Part model, mm, in its own coordinate system. Coordinates: 2 decimals unless noted, no trailing zeros. Order: outer loops, then holes, each group sorted by start corner. A loop starts at its lowest first (then second) coordinate and runs counter-clockwise, first axis right, second up.
1) Cut at B-B (y = 3.25). List the corners of the cut face in (x, z), and give its area (3 significant figures).
2) Cut at C-C (z = 45). Give the number of separate pieces and of enclosed holes in the cut face, and give its area (3 significant figures).
3) Wall check: L1, parallel to Y at x = 210.5, z = 0; L2, parallel to X at y = -0.5, z = 27.5. Give the ranges that are in metal, low to high.
4) Pin check, flat tips, straight feed: pin 1 Ø8 at (x, y) = (311.5, -3.5) entering from +Z; pin 2 Ø5 at (y, z) = (7.5, 44) entering from +X; pin 3 Ø6 at (x, y) = (398, -5.5) entering from -Z. Stop position of each tip, or through.
5) Cut at A-A (x = 258.5). List the corners of the cut face in (y, z), and give its area (3 significant figures).
Autodesk Inventor part; units mm, degrees
ref_plane "YZ Plane" through (0, 0, 0) normal (1, 0, 0) x (0, 1, 0)
ref_plane "XZ Plane" through (0, 0, 0) normal (0, 1, 0) x (-1, 0, 0)
ref_plane "XY Plane" through (0, 0, 0) normal (0, 0, 1) x (1, 0, 0)
sketch "Szkic1" plane through (0, 0, 0) normal (1, 0, 0) x (0, 1, 0)
  circle A0 centre (0, 0) radius 10
  dimension "d0" = 20
extrude "Wyciągnięcie proste1" add sketch "Szkic1" along normal blind 475
shell "Skorupa1" thickness 2 removed faces 2 at (475, -1.182, 3.1167) at (0, -1.182, 3.1167)
sketch "Szkic2" plane through (0, 0, 0) normal (0, 0, 1) x (1, 0, 0)
  line L0 (100, 28.3712) -> (100, -25.6691)
  line L1 (0, 10) -> (0, -10)
  point P0 (0, 0)
  dimension "d4" = 100
bend part "Gięcie części1" radius 50.9296 angle 45 line through (100, 28.3712, 0) along (0, -1, 0) centre toward (0, 0, 1) moving side (-1, 0, 0) both sides no
sketch "Szkic3" plane through (0, 0, 0) normal (0, 0, 1) x (1, 0, 0)
  line L0 (375, 37.2706) -> (375, -31.4113)
  line L1 (475, -10) -> (475, 10)
  point P0 (0, 0)
  dimension "d7" = 100
bend part "Gięcie części2" radius 50.9296 angle 45 line through (375, 37.2706, 0) along (0, -1, 0) centre toward (0, 0, 1) moving side (1, 0, 0) both sides no
sketch "Szkic4" plane through (0, 0, 0) normal (0, 1, 0) x (-1, 0, 0)
  line L0 (-446.368, 64.4144) -> (-460.5101, 50.2723) construction
  line L1 (-403.9416, 21.988) -> (-446.368, 64.4144) construction
  line L2 (-418.0837, 7.8459) -> (-460.5101, 50.2723) construction
  line L3 (-460.5101, 50.2723) -> (-446.368, 64.4144)
  line L4 (-446.368, 64.4144) -> (-432.2259, 50.2723)
  line L5 (-432.2259, 50.2723) -> (-460.5101, 50.2723)
  line L6 (-14.4899, 50.2723) -> (-28.632, 64.4144) construction
  line L7 (-28.632, 64.4144) -> (-71.0584, 21.988) construction
  line L8 (-14.4899, 50.2723) -> (-56.9163, 7.8459) construction
  line L9 (-14.4899, 50.2723) -> (-28.632, 64.4144)
  line L10 (-28.632, 64.4144) -> (-42.7741, 50.2723)
  line L11 (-42.7741, 50.2723) -> (-14.4899, 50.2723)
  point P0 (0, 0)
extrude "Wyciągnięcie proste2" cut sketch "Szkic4" along normal mid plane 20
equation "\"PromieńGięcia\" = Grubość"
equation "\"SzerokośćGięciaPodcięcia\" = Grubość"
equation "\"GłębokośćGięciaPodcięcia\" = 0.5 * Grubość"
equation "\"RozmiarPodcięciaNarożnika\" = 4 * Grubość"
equation "\"MinimalnaPozostałość\" = 2 * Grubość"
equation "\"PromieńPrzejścia\" = PromieńGięcia"
equation "\"Rozmiar_promienia_Jacobiego\" = PromieńGięcia"
equation "\"Wielk_odstępu\" = Grubość"
properties part number "Rura_barierka_oparcia" material "Aluminium AW-7020"
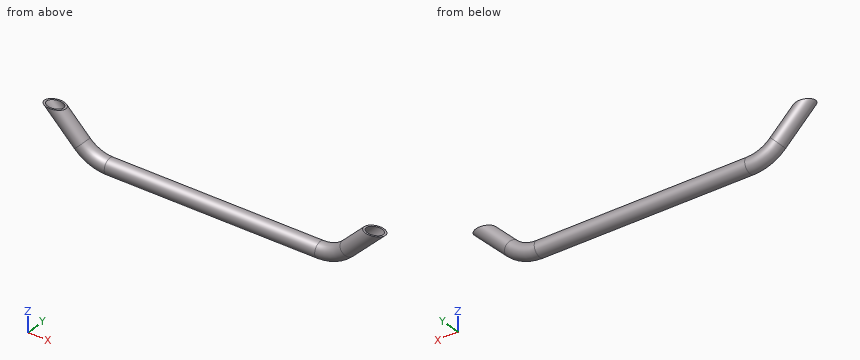
Geometry check:
1. outline: (15.26, 50.27) - (57.3, 8.23) arc R60.39 ccw to (100, -9.46) - (375, -9.46) arc R60.39 ccw to (417.7, 8.23) - (459.74, 50.27) - (456.71, 50.27) - (416.18, 9.75) arc R58.24 cw to (375, -7.31) - (100, -7.31) arc R58.24 cw to (58.82, 9.75) - (18.29, 50.27) - close; (38.97, 50.27) - (69.16, 20.09) arc R43.62 ccw to (100, 7.31) - (375, 7.31) arc R43.62 ccw to (405.84, 20.09) - (436.03, 50.27) - (432.99, 50.27) - (404.33, 21.6) arc R41.47 cw to (375, 9.46) - (100, 9.46) arc R41.47 cw to (70.67, 21.6) - (42.01, 50.27) - close
1. area: 1,950 mm2
2. separate pieces: 2
2. enclosed holes: 2
2. area: 320 mm2
3. L1: y = -10 to -8, 8 to 10
3. L2: x = 37.28 to 40.11, 62.7 to 65.53, 409.47 to 412.3, 434.89 to 437.72
4. pin 1: stops at z = 10
4. pin 2: stops at x = 453.45
4. pin 3: stops at z = -5.68
5. outline: circle Ø20 at (0, 0); hole circle Ø16 at (0, 0)
5. area: 113 mm2
